For this review, take the finished solid that the model builds, in its own axes (mm). A direction names the side the tool comes from. Give positions to 0.01 mm unless a question says otherwise; leave off trailing zeros. Loops run counter-clockwise (first coordinate to the right, second up) from the corner with the lowest first, then second, coordinate; pieces in that order, holes last.
```python
from build123d import *

# Parameters (mm, degrees)
F1_W          = 228.6
F1_H          = 50.8
F1_R          = 3.81
F2_DEPTH      = 6.35
F3_DEPTH      = 7.62
F5_DEPTH      = 25.4
F5_DEPTH_BACK = 25.4


with BuildPart() as f2:
    # F1 (on Front) → F2 (new body)
    with BuildSketch(Plane.XZ):
        with Locations((-0.0165204967, 25.4)):
            Rectangle(F1_W, F1_H)
        with Locations((-99.0765204967, 15.24)):
            Circle(F1_R, mode=Mode.SUBTRACT)
        with Locations((99.0434795033, 15.24)):
            Circle(F1_R, mode=Mode.SUBTRACT)
    extrude(amount=F2_DEPTH)

    # F0 (on Top) → F3 (join)
    with BuildSketch(Plane.XY):
        with BuildLine():
            Line((-114.3, 0), (0, 0))
            Line((0, 0), (114.3, 0))
            add(Edge.make_bspline(
                [(114.3, 0), (112.9042055321, 50.9900506367), (104.7924183286, 129.6019823877), (85.741828675, 158.2428378306), (76.2, 177.8)],
                knots=[0, 0, 0, 0, 0.604684, 1, 1, 1, 1], degree=3))
            Line((76.2, 177.8), (0, 177.8))
            Line((0, 177.8), (-76.2, 177.8))
            add(Edge.make_bspline(
                [(-114.3, 0), (-112.9042055321, 50.9900506367), (-104.7924183286, 129.6019823877), (-85.741828675, 158.2428378306), (-76.2, 177.8)],
                knots=[0, 0, 0, 0, 0.604684, 1, 1, 1, 1], degree=3))
        make_face()
    extrude(amount=F3_DEPTH)

    # F4 (on Right) → F5 (join, two sides)
    with BuildSketch(Plane.YZ) as f5_sk:
        Polygon((161.2199991941, 7.62), (0, 40.4569857569), (0, 7.62), align=None)
    extrude(amount=F5_DEPTH)
    extrude(f5_sk.sketch, amount=-F5_DEPTH_BACK)


solid = f2.part
```
Q1. Consider section A-A on z = 15.24. Give the boundary of the cut face in (x, y).
Answers:
outline: (-114.32, -6.35) - (-102.89, -6.35) - (-102.89, 0) - (-114.32, 0) - close; (-95.27, -6.35) - (95.23, -6.35) - (95.23, 0) - (25.4, 0) - (25.4, 123.81) - (-25.4, 123.81) - (-25.4, 0) - (-95.27, 0) - close; (102.85, -6.35) - (114.28, -6.35) - (114.28, 0) - (102.85, 0) - close
Q2. Consider section D-D on x = 54. Give the boundary of the cut face in (y, z).
Answers:
outline: (-6.35, 0) - (177.8, 0) - (177.8, 7.62) - (0, 7.62) - (0, 50.8) - (-6.35, 50.8) - close
Q3. For pin 1 Ø10 at (y, z) = (75, 16) entering from +X; pin 2 Ø6 at (x, y) = (89.5, 40) entering from -Z; pin 3 Ø6 at (x, y) = (0, 150) entering from +Z; pin 4 Ø10 at (y, z) = (78, 24.5) entering from -X, all flat-tipped, find the tip position at first contact; note any pin that passes through.
Answers:
pin 1: stops at x = 25.4
pin 2: stops at z = 0
pin 3: stops at z = 10.52
pin 4: stops at x = -25.4
Q4. Mouldability with a two-part tool opening along Z and no side actions: class faces 1 (the flat face through (-2, 87, 0)), 2 (the flat face through (0.36, 81.74, 23.81)), 3 (the cylindrical face through (102.68, -3.13, 16.38)) as +Z half, -Z half, draft (parallel to the pull), parting line (faces both ways), or undercut.
Answers:
face 1: -Z half
face 2: +Z half
face 3: undercut
Q5. Consider section B-B on x = 23. Give the boundary of the cut face in (y, z), plus the area to 3 significant figures.
Answers:
outline: (-6.35, 0) - (177.8, 0) - (177.8, 7.62) - (161.22, 7.62) - (0, 40.46) - (0, 50.8) - (-6.35, 50.8) - close
area: 4,320 mm2
Q6. For probe 1 along X at (y, z) = (-3, 15); probe 2 along Z at (x, y) = (-104.5, 48); probe 3 along Y at (x, z) = (12.5, 44.5), list the stretches that pass through material, from the lowest coordinate up.
Answers:
probe 1: x = -114.32 to -102.88, -95.27 to 95.24, 102.85 to 114.28
probe 2: z = 0 to 7.62
probe 3: y = -6.35 to 0
Q7. Machinability: for faces 4 (the flat face through (-25.4, 44, 17)), 5 (the flat face through (1, 177.8, 4)), 6 (the flat face through (-2, 0, 43)), 7 (the cylindrical face through (-95.44, -3.13, 16.38)), 8 (the flat face through (25.4, 44, 17)), which of the approach directions +Z, -Z, +X, -X, +Y, -Y give a long, thin tool a straight path to every point of the face, cutting with its end or side? Answer none if there is none.
Answers:
face 4: +Z, -X, +Y
face 5: +Z, -Z, +X, -X, +Y
face 6: +Z, +Y
face 7: +Y, -Y
face 8: +Z, +X, +Y
Q8. Consider section C-C on z = 34. Give the boundary of the cut face in (x, y), plus the area to 3 significant figures.
Answers:
outline: (-114.32, -6.35) - (114.28, -6.35) - (114.28, 0) - (25.4, 0) - (25.4, 31.7) - (-25.4, 31.7) - (-25.4, 0) - (-114.32, 0) - close
area: 3,060 mm2
